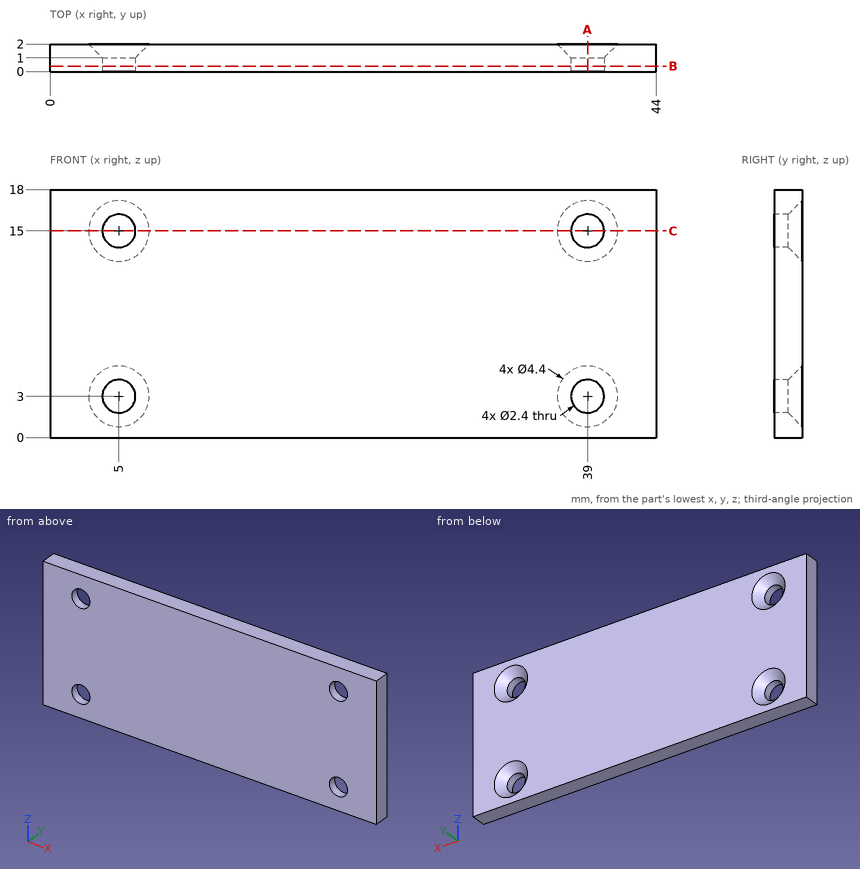
For this review, use the dimensioned drawing (mm, ordinates from the lowest corner) and the shaded views. Round coordinates to 2 decimals unless told otherwise and drop trailing zeros. Order: outer loops, then holes, each group sorted by start corner. A loop starts at its lowest first (then second) coordinate and runs counter-clockwise, first axis right, second up.
1) Consider section B-B (y = 0.4). State the section outline as (x, z) points.
The answers:
outline: (0, 0) - (44, 0) - (44, 18) - (0, 18) - close; hole circle Ø2.4 at (5, 3); hole circle Ø2.4 at (5, 15); hole circle Ø2.4 at (39, 3); hole circle Ø2.4 at (39, 15)
2) Consider section A-A (x = 39). State the section outline as (y, z) points.
The answers:
outline: (0, 0) - (2, 0) - (2, 0.8) - (1, 1.8) - (0, 1.8) - close; (0, 4.2) - (1, 4.2) - (2, 5.2) - (2, 12.8) - (1, 13.8) - (0, 13.8) - close; (0, 16.2) - (1, 16.2) - (2, 17.2) - (2, 18) - (0, 18) - close
3) For L1, parallel to X at y = 0.3, z = 3; L2, parallel to Z at x = 39, y = 0.65; L3, parallel to Z at x = 40.5, y = 1.9, list the stretches that pass through material, from the lowest coordinate up.
The answers:
L1: x = 0 to 3.8, 6.2 to 37.8, 40.2 to 44
L2: z = 0 to 1.8, 4.2 to 13.8, 16.2 to 18
L3: z = 0 to 1.53, 4.47 to 13.53, 16.47 to 18
4) Consider section C-C (z = 15). State the section outline as (x, y) points, plus the area to 3 significant figures.
The answers:
outline: (0, 0) - (3.8, 0) - (3.8, 1) - (2.8, 2) - (0, 2) - close; (6.2, 0) - (37.8, 0) - (37.8, 1) - (36.8, 2) - (7.2, 2) - (6.2, 1) - close; (40.2, 0) - (44, 0) - (44, 2) - (41.2, 2) - (40.2, 1) - close
area: 76.4 mm2
5) Clearance check with a flat-ended pin moving along its axis: pin 1 Ø4 at (x, z) = (5, 15) entering from +Y. State where the tip first meets the part, or that it passes through.
The answers:
pin 1: stops at y = 1.8
